Geometry: see drawing. Coordinates: mm, zero at the bounding-box minimum. A direction names the side the tool comes from. Coordinates: 2 decimals unless noted, no trailing zeros. Loops run counter-clockwise (first coordinate to the right, second up) from the corner with the lowest first, then second, coordinate; pieces in that order, holes last. Notation, with made-up numbers: (69.25, -15.75) - (112.25, -15.75) arc R13 cw to (112.25, 1.25) - close; hole circle Ø4 at (-37, 34). An arc over 180 degrees is marked (long way). Answer in a Markdown table with one row per item.
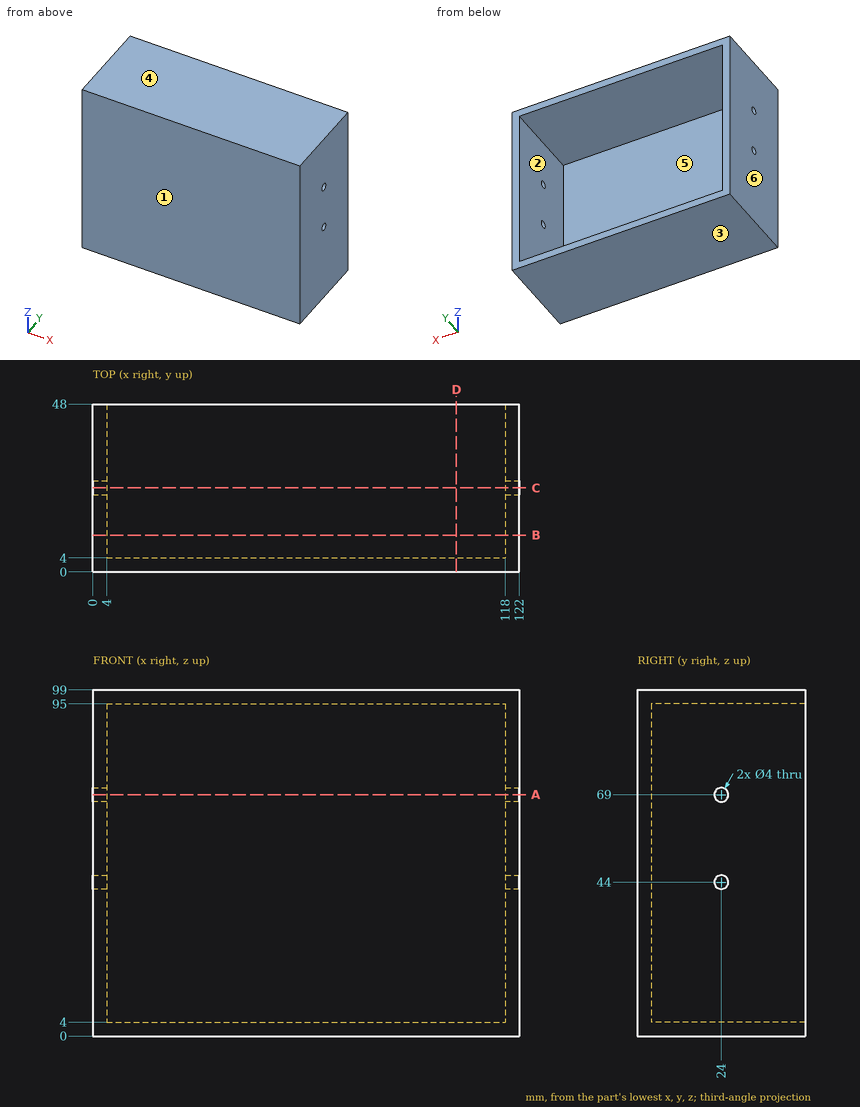
(1) Cut plane D-D on x = 104. Output: boundary loops of the cut face in (y, z), then the cut area to 3 significant figures.
Verdict:
| item | result |
|---|---|
| outline | (0, 0) - (48, 0) - (48, 4) - (4, 4) - (4, 95) - (48, 95) - (48, 99) - (0, 99) - close |
| area | 748 mm² |
(2) First-contact query: pin 1 Ø10 at (x, z) = (52.5, 43) entering from +Y. Flat tip, straight axial feed; report the tip coordinate or a pass-through.
Verdict:
| item | result |
|---|---|
| pin 1 | stops at y = 4 |
(3) Cut plane A-A on z = 69. Output: boundary loops of the cut face in (x, y), then the cut area to 3 significant figures.
Verdict:
| item | result |
|---|---|
| outline | (0, 0) - (122, 0) - (122, 22) - (118, 22) - (118, 4) - (4, 4) - (4, 22) - (0, 22) - close; (0, 26) - (4, 26) - (4, 48) - (0, 48) - close; (118, 26) - (122, 26) - (122, 48) - (118, 48) - close |
| area | 808 mm² |
(4) Ray query, probe 1 along X at (y, z) = (42.5, 75); probe 2 along Z at (x, y) = (49, 28); probe 3 along Y at (x, z) = (2.15, 44). Return the intervals inside material, ascending.
Verdict:
| item | result |
|---|---|
| probe 1 | x = 0 to 4, 118 to 122 |
| probe 2 | z = 0 to 4, 95 to 99 |
| probe 3 | y = 0 to 22, 26 to 48 |
(5) Cut plane B-B on y = 10.5. Output: boundary loops of the cut face in (x, z).
Verdict:
| item | result |
|---|---|
| outline | (0, 0) - (122, 0) - (122, 99) - (0, 99) - close; hole (4, 4) - (118, 4) - (118, 95) - (4, 95) - close |
(6) Pull-direction query (Z, two-part tool) for the marked faces 1, 2, 3 and 4; classes: pulls with the +Z half, pulls with the -Z half, needs draft (parallel to the pull), parting line crosses it, or undercut.
Verdict:
| item | result |
|---|---|
| face 1 | needs draft |
| face 2 | undercut |
| face 3 | pulls with the -Z half |
| face 4 | pulls with the +Z half |
(7) Access query for the marked faces 5 and 6. Directions: +Z, -Z, +X, -X, +Y, -Y. A direction counts if a zero-diameter tool reaches every point of the face in a straight line with its end or side. Return the directions, or none.
Verdict:
| item | result |
|---|---|
| face 5 | +Y |
| face 6 | +Z, -Z, -X, +Y, -Y |
(8) Cut plane C-C on y = 24. Output: boundary loops of the cut face in (x, z), then the cut area to 3 significant figures.
Verdict:
| item | result |
|---|---|
| outline | (0, 0) - (122, 0) - (122, 42) - (118, 42) - (118, 4) - (4, 4) - (4, 42) - (0, 42) - close; (0, 46) - (4, 46) - (4, 67) - (0, 67) - close; (0, 71) - (4, 71) - (4, 95) - (118, 95) - (118, 71) - (122, 71) - (122, 99) - (0, 99) - close; (118, 46) - (122, 46) - (122, 67) - (118, 67) - close |
| area | 1,640 mm² |
